Drawing for the job (mm, zero at the part's lowest x, y, z). Round coordinates to 2 decimals unless told otherwise and drop trailing zeros. Write each loop counter-clockwise with the first axis right and the second up, starting at its lowest first coordinate (ties: lowest second). Pieces come first, ordered by that corner, then holes. Notation, with made-up numbers: M 82,49.25 L 102,49.25 A35 ccw 102,88.25 Z; hole C 48,53.5 d4. An arc over 180 degrees is marked long. Use a Markdown table: item, result. Add a question column.
1) Wall check: probe 1 along X at (y, z) = (55, 6); probe 2 along Z at (x, y) = (471, 53); probe 3 along X at (y, z) = (159, 103). Give the ranges that are in metal, low to high.
2) Two-plate mould, pull along X, no slides. Class the marked faces 1, 2 and 3: released by +X, released by -X, zero draft, split by the parting line, or undercut.
3) Drop flat-ended pins along their axis: P1, Ø22, axis at y = 235.5, z = 107, coming from the +X side; P2, Ø6, axis at x = 185.5, z = 110, coming from the +Y side; P3, Ø10, axis at y = 173, z = 110, coming from the -X side; P4, Ø4, axis at x = 414, y = 302.5, coming from the -Z side. Give the stop position or say it passes through.
4) Slice it at B-B on y = 281. Write the cut outline in (x, z).
5) Slice it at A-A on z = 26.5. Write the cut outline in (x, y).
6) Slice it at C-C on x = 357.5. Write the cut outline in (y, z).
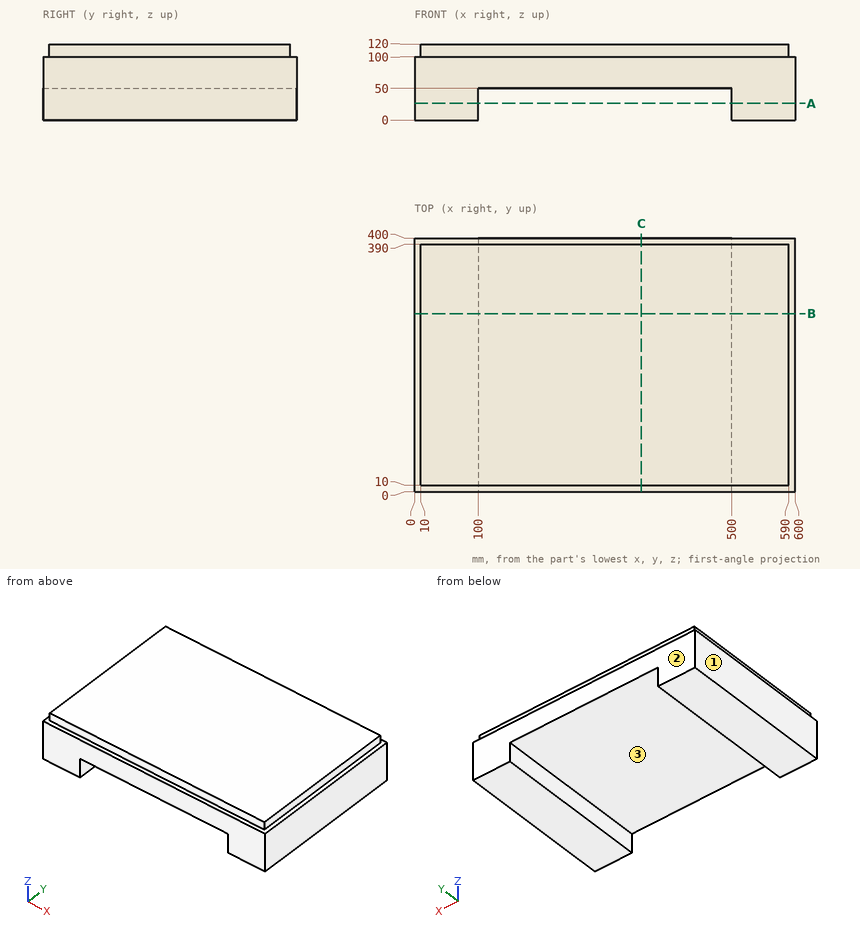
Entries:
| question | item | result |
|---|---|---|
| 1 | probe 1 | x = 0 to 100, 500 to 600 |
| 1 | probe 2 | z = 50 to 120 |
| 1 | probe 3 | x = 10 to 590 |
| 2 | face 1 | released by -X |
| 2 | face 2 | zero draft |
| 2 | face 3 | undercut |
| 3 | P1 | stops at x = 600 |
| 3 | P2 | stops at y = 390 |
| 3 | P3 | stops at x = 10 |
| 3 | P4 | stops at z = 50 |
| 4 | outline | M 0,0 L 100,0 L 100,50 L 500,50 L 500,0 L 600,0 L 600,100 L 590,100 L 590,120 L 10,120 L 10,100 L 0,100 Z |
| 5 | outline | M 0,0 L 100,0 L 100,400 L 0,400 Z; M 500,0 L 600,0 L 600,400 L 500,400 Z |
| 6 | outline | M 0,50 L 400,50 L 400,100 L 390,100 L 390,120 L 10,120 L 10,100 L 0,100 Z |
